The model under review builds one solid part; all positions refer to its coordinate system, in mm. Coordinates: 2 decimals unless noted, no trailing zeros. Order: outer loops, then holes, each group sorted by start corner. A loop starts at its lowest first (then second) coordinate and runs counter-clockwise, first axis right, second up.
```python
from build123d import *

# Parameters (mm, degrees)
F0_R     = 225
F1_DEPTH = 150
F2_R     = 50
F4_D     = 100


with BuildPart() as f1:
    # F0 (on Front) → F1 (new body)
    with BuildSketch(Plane.XZ):
        Circle(F0_R)
    extrude(amount=F1_DEPTH)

    # F2
    f2_edges = [f1.edges().sort_by_distance(p)[0] for p in [
        (-225, -150, 0),
        (-225, 0, 0),
    ]]
    fillet(f2_edges, radius=F2_R)

    # F4 (through all)
    with Locations(Plane.XZ.offset(150)):
        with Locations((0, 0)):
            Hole(F4_D / 2)


solid = f1.part
```
(1) We need section B-B, the plane z = 0. Write out the cut boundary in (x, y).
A:
outline: (-225, -100) arc R50 ccw to (-175, -150) - (-50, -150) - (-50, 0) - (-175, 0) arc R50 ccw to (-225, -50) - close; (50, -150) - (175, -150) arc R50 ccw to (225, -100) - (225, -50) arc R50 ccw to (175, 0) - (50, 0) - close
(2) We need section D-D, the plane y = -30.5. Write out the cut boundary in (x, z), and give its area (3 significant figures).
A:
outline: circle Ø442.08 at (0, 0); hole circle Ø100 at (0, 0)
area: 146,000 mm2
(3) For pin 1 Ø5 at (x, z) = (-167.5, 121) entering from +Y; pin 2 Ø12 at (x, y) = (-96, -75.5) entering from +Z; pin 3 Ø5 at (y, z) = (-39, -63) entering from -X, all flat-tipped, find the tip position at first contact; note any pin that passes through.
A:
pin 1: stops at y = -9.36
pin 2: stops at z = 206.22
pin 3: stops at x = -215.63
(4) Draft analysis for pull direction Z (two halves, no side actions). For faces 1 (the face through (36, -150, -36)), 2 (the face through (-47.69, -73.95, 15.02)), 3 (the face through (-224.782, -74.65, 9.893)), state which applies: released by +Z, released by -Z, zero draft, split by the parting line, or undercut.
A:
face 1: zero draft
face 2: undercut
face 3: split by the parting line
(5) We need section A-A, the plane x = 0. Write out the cut boundary in (y, z).
A:
outline: (-150, -175) arc R50 ccw to (-100, -225) - (-50, -225) arc R50 ccw to (0, -175) - (0, -50) - (-150, -50) - close; (-150, 50) - (0, 50) - (0, 175) arc R50 ccw to (-50, 225) - (-100, 225) arc R50 ccw to (-150, 175) - close
(6) Wall thickness on probe 1 along Z at (x, y) = (0, -78); probe 2 along Z at (x, y) = (0, -37.5); probe 3 along X at (y, z) = (-73.5, 9): over which ranges is each line inside the solid? List them lowest first.
A:
probe 1: z = -225 to -50, 50 to 225
probe 2: z = -223.41 to -50, 50 to 223.41
probe 3: x = -224.82 to -49.18, 49.18 to 224.82
(7) We need section C-C, the plane y = -76. Write out the cut boundary in (x, z), and give its area (3 significant figures).
A:
outline: circle Ø450 at (0, 0); hole circle Ø100 at (0, 0)
area: 151,000 mm2
